Read the model definition and answer for the solid it produces. Units are mm, in the model's axes. A direction names the side the tool comes from. Round coordinates to 2 decimals unless told otherwise and drop trailing zeros. Order: outer loops, then holes, each group sorted by start corner. A loop starts at its lowest first (then second) coordinate and runs counter-clockwise, first axis right, second up. Notation, with made-up numbers: (76, 12) - (89, 12) arc R19 ccw to (89, 18) - close; hole circle Ø11 at (41.5, 11.5). An arc over 180 degrees is marked (long way). Answer as a JSON object with one key per item and string values. Group by question number.
Q1. A cutting plane is placed at B-B on z = 0. Determine the outline of the cut face in (x, y), and give its area (3 significant figures).
Q2. A cutting plane is placed at C-C on x = 19.25. Determine the outline of the cut face in (y, z).
Q3. A cutting plane is placed at D-D on x = 1.5. Determine the outline of the cut face in (y, z), and give its area (3 significant figures).
Q4. A tool of negligible diameter and unlimited length cuts with its end or side. For faces 4 (the cylindrical face through (16.67, -3.735, -10.638)), 5 (the flat face through (11, 4, -3)), 6 (the flat face through (5, 0, 8)), 7 (the flat face through (5.01, 14.24, -0.87)), from which of +Z, -Z, +X, -X, +Y, -Y can it reach the whole face along a straight path? Write none if from no direction.
Q5. Consider line 1 (Z direction, x = 5.5, y = 0); line 2 (Z direction, x = 3, y = 0); line 3 (X direction, y = 0, z = 4.9). Determine where each line is inside the solid, lowest interval first.
Q6. The mould has two halves that part along Y. Classify faces 1 (the flat face through (4.99, -0.86, 14.24)), 2 (the flat face through (4.5, 14, 0)), 3 (the cylindrical face through (16.67, 3.735, 10.638)): pulls with the +Y half, pulls with the -Y half, needs draft (parallel to the pull), parting line crosses it, or undercut.
Q7. Given pin 1 Ø1 at (x, y) = (5.5, 0) entering from +Z; pin 2 Ø8 at (x, z) = (9, 8) entering from -Y; pin 3 Ø3.5 at (x, y) = (5.5, 0) entering from +Z; pin 4 Ø1 at (x, z) = (5.5, 0.5) entering from +Y, each flat-ended and moving along its own axis, determine where each tip first touches the part or whether it passes through.
Autodesk Inventor part; units mm, degrees
ref_plane "part1a_XY" through (0, 0, 0) normal (1, 0, 0) x (0, 0, -1)
ref_plane "part1a_YZ" through (0, 0, 0) normal (0, 0, -1) x (0, 1, 0)
ref_plane "part1a_ZX" through (0, 0, 0) normal (0, 1, 0) x (1, 0, 0)
sketch "Sketch_1" plane through (0, 0, 0) normal (0, 0, 1) x (1, 0, 0)
  line L0 (22.5, 0) -> (0, 0)
  line L1 (0, 14.5) -> (0, 4)
  line L2 (0, 4) -> (22.5, 4)
  line L3 (22.5, 4) -> (22.5, 14)
  line L4 (22.5, 14) -> (21.5, 15)
  line L5 (21.5, 15) -> (0.5, 15)
  line L6 (0.5, 15) -> (0, 14.5)
revolve "Revolution1" add sketch "Sketch_1" angle 360 about axis through (22.5, 0, 0) along (1, 0, 0)
sketch "Sketch_2" plane through (11, 0, 0) normal (1, 0, 0) x (0, 0, -1)
  arc A0 (-13.4651, -6.61) -> (13.4651, -6.61) centre (0, 0) ccw
  arc A1 (13.4651, -6.61) -> (7.3157, -1.6525) centre (0, -17.0197) ccw
  arc A2 (7.3157, -1.6525) -> (7.3157, 1.6525) centre (0, 0) ccw
  arc A3 (7.3157, 1.6525) -> (13.4651, 6.61) centre (0, 17.0197) ccw
  arc A4 (13.4651, 6.61) -> (-13.4651, 6.61) centre (0, 0) ccw
  arc A5 (-13.4651, 6.61) -> (-7.3157, 1.6525) centre (0, 17.0197) ccw
  arc A6 (-7.3157, 1.6525) -> (-7.3157, -1.6525) centre (0, 0) ccw
  arc A7 (-7.3157, -1.6525) -> (-13.4651, -6.61) centre (0, -17.0197) ccw
extrude "Extrusion1" cut sketch "Sketch_2" along normal blind 11.5
sketch "Sketch_7" plane through (0, 0, 0) normal (0, 0, 1) x (1, 0, 0)
  line L0 (5.5, 0) -> (5.5, 15)
  line L1 (5.5, 15) -> (7.5, 15)
  line L2 (7.5, 15) -> (7.121, 14.621)
  line L3 (7.121, 14.621) -> (7.121, 0.379)
  line L4 (7.121, 0.379) -> (7.5, 0)
  line L5 (7.5, 0) -> (5.5, 0)
  line L6 (5.5, 0) -> (5.5, 15)
revolve "Revolution2" cut sketch "Sketch_7" angle 360 about axis through (5.5, 0, 0) along (0, -1, 0)
sketch "Sketch_8" plane through (0, 0, 0) normal (0, 1, 0) x (-1, 0, 0)
  line L0 (-5.5, 15) -> (-5.5, 0)
  line L1 (-5.5, 0) -> (-7.5, 0)
  line L2 (-7.5, 0) -> (-7.121, 0.379)
  line L3 (-7.121, 0.379) -> (-7.121, 14.621)
  line L4 (-7.121, 14.621) -> (-7.5, 15)
  line L5 (-7.5, 15) -> (-5.5, 15)
  line L6 (-5.5, 15) -> (-5.5, 0)
revolve "Revolution3" cut sketch "Sketch_8" angle 360 about axis through (5.5, 0, 15) along (0, 0, 1)
sketch "Sketch_12" plane through (0, 0, 0) normal (0, 0, 1) x (1, 0, 0)
  line L0 (5.5, 8) -> (5.5, 15)
  line L1 (5.5, 15) -> (7.0705, 15)
  line L2 (7.0705, 15) -> (7.5, 14.5705)
  line L3 (7.5, 14.5705) -> (7.5, 8.4295)
  line L4 (7.5, 8.4295) -> (7.0705, 8)
  line L5 (7.0705, 8) -> (5.5, 8)
  line L6 (5.5, 8) -> (5.5, 15)
revolve "Revolution4" add sketch "Sketch_12" angle 360 about axis through (5.5, 8, 0) along (0, -1, 0)
sketch "Sketch_13" plane through (0, 0, 0) normal (0, 1, 0) x (-1, 0, 0)
  line L0 (-5.5, 15) -> (-5.5, 8)
  line L1 (-5.5, 8) -> (-7.0705, 8)
  line L2 (-7.0705, 8) -> (-7.5, 8.4295)
  line L3 (-7.5, 8.4295) -> (-7.5, 14.5705)
  line L4 (-7.5, 14.5705) -> (-7.0705, 15)
  line L5 (-7.0705, 15) -> (-5.5, 15)
  line L6 (-5.5, 15) -> (-5.5, 8)
revolve "Revolution5" add sketch "Sketch_13" angle 360 about axis through (5.5, 0, 15) along (0, 0, 1)
sketch "Sketch_14" plane through (0, 13.5, 0) normal (0, 1, 0) x (1, 0, 0)
  line L0 (4.5, -0.5774) -> (5.5, -1.1547)
  line L1 (5.5, -1.1547) -> (6.5, -0.5774)
  line L2 (6.5, -0.5774) -> (6.5, 0.5774)
  line L3 (6.5, 0.5774) -> (5.5, 1.1547)
  line L4 (5.5, 1.1547) -> (4.5, 0.5774)
  line L5 (4.5, 0.5774) -> (4.5, -0.5774)
extrude "Extrusion2" cut sketch "Sketch_14" along normal blind 1.5
sketch "Sketch_15" plane through (0, 0, 13.5) normal (0, 0, 1) x (1, 0, 0)
  line L0 (4.5, -0.5774) -> (5.5, -1.1547)
  line L1 (5.5, -1.1547) -> (6.5, -0.5774)
  line L2 (6.5, -0.5774) -> (6.5, 0.5774)
  line L3 (6.5, 0.5774) -> (5.5, 1.1547)
  line L4 (5.5, 1.1547) -> (4.5, 0.5774)
  line L5 (4.5, 0.5774) -> (4.5, -0.5774)
extrude "Extrusion3" cut sketch "Sketch_15" along normal blind 1.5
ref_plane "part1a_XY" through (0, 0, 0) normal (1, 0, 0) x (0, 0, -1)
ref_plane "part1a_YZ" through (0, 0, 0) normal (0, 0, -1) x (0, 1, 0)
ref_plane "part1a_ZX" through (0, 0, 0) normal (0, 1, 0) x (1, 0, 0)
ref_plane "part1b_XY" through (12.5, 0, 0) normal (1, 0, 0) x (0, 0, -1)
ref_plane "part1b_YZ" through (12.5, 0, 0) normal (0, 0, -1) x (0, 1, 0)
ref_plane "part1b_ZX" through (12.5, 0, 0) normal (0, 1, 0) x (1, 0, 0)
ref_plane "part1c_XY" through (22.5, 0, 0) normal (1, 0, 0) x (0, 0, -1)
ref_plane "part1c_YZ" through (22.5, 0, 0) normal (0, 0, -1) x (0, 1, 0)
ref_plane "part1c_ZX" through (22.5, 0, 0) normal (0, 1, 0) x (1, 0, 0)
properties part number "MJT-30-BL-8-12 Hub 1"
Result set:
{
 "1": {"outline": "(0, -14.5) - (0.5, -15) - (11, -15) - (11, -4) - (0, -4) - close; (0, 4) - (3.88, 4) - (3.88, 8.05) - (3.93, 8) - (7.07, 8) - (7.12, 8.05) - (7.12, 4) - (11, 4) - (11, 15) - (7.5, 15) - (7.29, 14.79) - (7.07, 15) - (6.5, 15) - (6.5, 13.5) - (4.5, 13.5) - (4.5, 15) - (3.93, 15) - (3.71, 14.79) - (3.5, 15) - (0.5, 15) - (0, 14.5) - close", "area": "226 mm²"},
 "2": {"outline": "(-6.61, -13.47) arc R15 ccw to (6.61, -13.47) arc R17.02 cw to (1.65, -7.32) arc R7.5 cw to (-1.65, -7.32) arc R17.02 cw to start; (-6.61, 13.47) arc R17.02 cw to (-1.65, 7.32) arc R7.5 cw to (1.65, 7.32) arc R17.02 cw to (6.61, 13.47) arc R15 ccw to start"},
 "3": {"outline": "circle Ø30 at (0, 0); hole circle Ø8 at (0, 0)", "area": "657 mm²"},
 "4": {"face 4": "+X, -Y", "face 5": "+X", "face 6": "none", "face 7": "+Y"},
 "5": {"line 1": "z = -15 to -4, 8 to 13.5", "line 2": "z = -15 to -4, 4 to 15", "line 3": "x = 0 to 3.88, 7.12 to 11"},
 "6": {"face 1": "undercut", "face 2": "needs draft", "face 3": "pulls with the +Y half"},
 "7": {"pin 1": "stops at z = 13.5", "pin 2": "stops at y = -14.46", "pin 3": "stops at z = 15", "pin 4": "stops at y = 13.5"}
}
